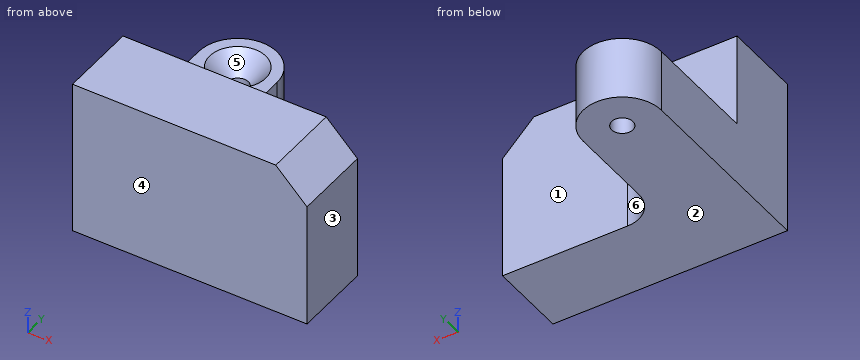
```python
from build123d import *

# Parameters (mm, degrees)
F0_W           = 12.7
F0_H           = 19.05
F1_DEPTH       = 25.4
F2_DEPTH       = 15.24
F3_D           = 3.4544
F3_START       = 15.24
F3_CSINK_D     = 9.1186
F3_CSINK_ANGLE = 82
F4_R           = 5.08
F5_SIZE        = 5.08


with BuildPart() as f1:
    # F0 (on Top) → F1 (new body)
    with BuildSketch(Plane.XY):
        Polygon((-19.05, 6.35), (-19.05, -6.35), (19.05, -6.35), (19.05, 6.35), (-6.35, 6.35), align=None)
        with Locations((-12.7, 15.875)):
            Rectangle(F0_W, F0_H)
        with BuildLine():
            ThreePointArc((-6.35, 25.4), (-12.7, 31.75), (-19.05, 25.4))
            Line((-19.05, 25.4), (-6.35, 25.4))
        make_face()
    extrude(amount=-F1_DEPTH)

    # F0 (on Top) → F2 (cut)
    with BuildSketch(Plane.XY):
        with Locations((-12.7, 15.875)):
            Rectangle(F0_W, F0_H)
        with BuildLine():
            ThreePointArc((-6.35, 25.4), (-12.7, 31.75), (-19.05, 25.4))
            Line((-19.05, 25.4), (-6.35, 25.4))
        make_face()
    extrude(amount=-F2_DEPTH, mode=Mode.SUBTRACT)

    # F3 (through all)
    # its depths count from where the whole tool has entered the part; down to there all is cleared
    with Locations(Plane.XY.offset(-F3_START)):
        with Locations((-12.7, 25.4)):
            CounterSinkHole(F3_D / 2, F3_CSINK_D / 2, counter_sink_angle=F3_CSINK_ANGLE)

    # F4
    f4_edges = [f1.edges().sort_by_distance(p)[0] for p in [
        (-6.35, 6.35, -20.32),
    ]]
    fillet(f4_edges, radius=F4_R)

    # F5
    f5_edges = [f1.edges().sort_by_distance(p)[0] for p in [
        (19.05, 0, 0),
    ]]
    chamfer(f5_edges, length=F5_SIZE)


solid = f1.part
```
Model file for the job. Use its own axes, mm. Face numbers are marked on the shaded views. A direction names the side the tool comes from. Coordinates: 2 decimals unless noted, no trailing zeros. Loops run counter-clockwise (first coordinate to the right, second up) from the corner with the lowest first, then second, coordinate; pieces in that order, holes last. Notation, with made-up numbers: (-22, -18) - (-15, -18) arc R26 cw to (-15, 9) - close; hole circle Ø5 at (89, 30.25). An arc over 180 degrees is marked (long way). Write item = value, one per line. Start each with the question number.
Item 1: Saw through at D-D, the plane x = -5. List the corners of the cut face in (y, z).
Item 2: Saw through at A-A, the plane x = -12.7. List the corners of the cut face in (y, z).
Item 3: Saw through at B-B, the plane z = -12.5. List the corners of the cut face in (x, y), then the cut area to 3 significant figures.
Item 4: Wall check: probe 1 along Y at (x, z) = (-12.7, -22); probe 2 along X at (y, z) = (25.4, -22); probe 3 along Y at (x, z) = (-8, -8.25). Give the ranges that are in metal, low to high. Write a range as [from, to].
Item 5: 3-axis set-ups, long thin cutter, end or side, ignore diameter. For the marked faces 1 and 2: which of +Z, -Z, +X, -X, +Y, -Y reach the whole face in a straight line?
Item 6: Drop flat-ended pins along their axis: pin 1 Ø5 at (x, z) = (1, -12.5) entering from +Y; pin 2 Ø12 at (y, z) = (11, -14) entering from -X; pin 3 Ø1.5 at (y, z) = (8.5, -17) entering from +X; pin 4 Ø6 at (x, z) = (1.5, -15) entering from +Y. Give the stop position or say it passes through.
Item 7: Pull direction Y, two halves, no side cores. Call the marked faces 3, 4, 5 and 6: +Y half, -Y half, draft (parallel to the pull), parting line (faces both ways), or undercut.
Item 8: Saw through at C-C, the plane x = 1. List the corners of the cut face in (y, z).
Answers:
q1.outline = (-6.35, -25.4) - (7.98, -25.4) - (7.98, -15.24) - (6.35, -15.24) - (6.35, 0) - (-6.35, 0) - close
q2.outline = (-6.35, -25.4) - (23.67, -25.4) - (23.67, -18.5) - (20.84, -15.24) - (6.35, -15.24) - (6.35, 0) - (-6.35, 0) - close; (27.13, -25.4) - (31.75, -25.4) - (31.75, -15.24) - (29.96, -15.24) - (27.13, -18.5) - close
q3.outline = (-19.05, -6.35) - (19.05, -6.35) - (19.05, 6.35) - (-19.05, 6.35) - close
q3.area = 484 mm2
q4.probe_1 = [-6.35, 23.67], [27.13, 31.75]
q4.probe_2 = [-19.05, -14.43], [-10.97, -6.35]
q4.probe_3 = [-6.35, 6.35]
q5.face_1 = +Z, +X, +Y
q5.face_2 = -Z, +X, -X, +Y, -Y
q6.pin_1 = 6.35
q6.pin_2 = -19.05
q6.pin_3 = -4.77
q6.pin_4 = 6.35
q7.face_3 = draft
q7.face_4 = -Y half
q7.face_5 = undercut
q7.face_6 = +Y half
q8.outline = (-6.35, -25.4) - (6.35, -25.4) - (6.35, 0) - (-6.35, 0) - close
